```python
from build123d import *

# Parameters (mm, degrees)
F0_W         = 45
F0_H         = 45
F1_DEPTH     = 2
F2_R         = 8
F3_DEPTH     = 25
F4_W         = 23
F4_H         = 3.9995294809
F4_H_2       = 4
F5_DEPTH     = 9.8
F6_W         = 23
F6_H         = 9
F6_H_2       = 4
F7_DEPTH     = 2
F8_W         = 23
F8_H         = 13
F9_DEPTH     = 2
F10_W        = 2
F10_H        = 45
F11_DEPTH    = 7.7
F12_W        = 7
F12_H        = 45
F13_W        = 7
F13_H        = 45
F14_DEPTH    = 2
F15_T1_DEPTH = 23
F15_T3_DEPTH = 45


# Not quite as in the source:
# - a fillet or chamfer that OpenCascade refuses, or shapes differently, is made with other operations: its cross-section is extruded or revolved along the edge and cut away or added


with BuildPart() as f1:
    # F0 (on Top) → F1 (new body)
    with BuildSketch(Plane.XY):
        Rectangle(F0_W, F0_H)
    extrude(amount=F1_DEPTH)

    # F2 (on face) → F3 (cut)
    with BuildSketch(Plane.XY.offset(2)):
        Circle(F2_R)
    extrude(amount=-F3_DEPTH, mode=Mode.SUBTRACT)

    # F4 (on face) → F5 (join)
    with BuildSketch(Plane.XY.offset(2)):
        with Locations((0, 22.5)):
            Rectangle(F4_W, F4_H)
        with Locations((0, -22.5)):
            Rectangle(F4_W, F4_H_2)
    extrude(amount=-F5_DEPTH)

    # F6 (on face) → F7 (join)
    with BuildSketch(Plane(origin=(0, 0, -7.8), x_dir=(1, 0, 0), z_dir=(0, 0, -1))):
        with Locations((0, 16)):
            Rectangle(F6_W, F6_H)
        with Locations((0, 22.5)):
            Rectangle(F6_W, F6_H_2)
    extrude(amount=F7_DEPTH)

    # F8 (on face) → F9 (join)
    with BuildSketch(Plane(origin=(0, 0, -7.8), x_dir=(1, 0, 0), z_dir=(0, 0, -1))):
        with Locations((0, -17.9997647405)):
            Rectangle(F8_W, F8_H)
    extrude(amount=F9_DEPTH)

    # F10 (on face) → F11 (join)
    with BuildSketch(Plane(origin=(0, 0, 0), x_dir=(1, 0, 0), z_dir=(0, 0, -1))):
        with Locations((-21.5, 0)):
            Rectangle(F10_W, F10_H)
        with Locations((21.5, 0)):
            Rectangle(F10_W, F10_H)
    extrude(amount=F11_DEPTH)

    # F12 (on face) + F13 (on face) → F14 (join)
    with BuildSketch(Plane(origin=(0, 0, -7.7), x_dir=(1, 0, 0), z_dir=(0, 0, -1))):
        with Locations((-24, 0)):
            Rectangle(F12_W, F12_H)
    with BuildSketch(Plane(origin=(0, 0, -7.7), x_dir=(1, 0, 0), z_dir=(0, 0, -1))):
        with Locations((24, 0)):
            Rectangle(F13_W, F13_H)
    extrude(amount=F14_DEPTH)

    # F15: fillet of radius 5 on 8 edges, made by hand

    # F15_s2 → F15_t1 (join)
    with BuildSketch(Plane.YZ.offset(-11.5)):
        with BuildLine():
            ThreePointArc((-15.5, -7.8), (-19.0355339059, -6.3355339059), (-20.5, -2.8))
            Line((-20.5, -2.8), (-20.5, -7.8))
            Line((-20.5, -7.8), (-15.5, -7.8))
        make_face()
        with BuildLine():
            ThreePointArc((15.5002352595, -7.8), (19.0357691655, -6.3355339059), (20.5002352595, -2.8))
            Line((20.5002352595, -2.8), (20.5002352595, -7.8))
            Line((20.5002352595, -7.8), (15.5002352595, -7.8))
        make_face()
        with BuildLine():
            ThreePointArc((20.5002352595, -5), (19.0357691655, -1.4644660941), (15.5002352595, 0))
            Line((15.5002352595, 0), (20.5002352595, 0))
            Line((20.5002352595, 0), (20.5002352595, -5))
        make_face()
        with BuildLine():
            ThreePointArc((-20.5, -5), (-19.0355339059, -1.4644660941), (-15.5, 0))
            Line((-15.5, 0), (-20.5, 0))
            Line((-20.5, 0), (-20.5, -5))
        make_face()
    extrude(amount=F15_T1_DEPTH)

    # F15_s4 → F15_t3 (join)
    with BuildSketch(Plane.XZ.offset(-22.5)):
        with BuildLine():
            ThreePointArc((20.5, -5), (19.0355339059, -1.4644660941), (15.5, 0))
            Line((15.5, 0), (20.5, 0))
            Line((20.5, 0), (20.5, -5))
        make_face()
        with BuildLine():
            ThreePointArc((-20.5, -5), (-19.0355339059, -1.4644660941), (-15.5, 0))
            Line((-15.5, 0), (-20.5, 0))
            Line((-20.5, 0), (-20.5, -5))
        make_face()
        with BuildLine():
            ThreePointArc((-22.5, -2.7), (-23.9644660941, -6.2355339059), (-27.5, -7.7))
            Line((-27.5, -7.7), (-22.5, -7.7))
            Line((-22.5, -7.7), (-22.5, -2.7))
        make_face()
        with BuildLine():
            ThreePointArc((27.5, -7.7), (23.9644660941, -6.2355339059), (22.5, -2.7))
            Line((22.5, -2.7), (22.5, -7.7))
            Line((22.5, -7.7), (27.5, -7.7))
        make_face()
    extrude(amount=F15_T3_DEPTH)


solid = f1.part
```
Input: part model. Units: mm. Frame: model coordinates. A direction names the side the tool comes from. Give positions to 0.01 mm unless a question says otherwise; leave off trailing zeros. Order: outer loops, then holes, each group sorted by start corner. A loop starts at its lowest first (then second) coordinate and runs counter-clockwise, first axis right, second up.
1. Line query: probe 1 along X at (y, z) = (-13.5, -8); probe 2 along Z at (x, y) = (7, -15); probe 3 along Y at (x, z) = (0, 1.1). Output: solid intervals per line, ascending.
Computed:
probe 1: x = -27.5 to -20.5, -11.5 to 11.5, 20.5 to 27.5
probe 2: z = -9.8 to -7.8, 0 to 2
probe 3: y = -24.5 to -8, 8 to 24.5
2. Draft query along X for faces 1 (the face through (27.5, 0, -9)), 2 (the face through (0, 24.5, -4)), 3 (the face through (-23.93, 0.32, -6.2)), 4 (the face through (-19.07, 0.32, -1.5)). Return one class per face: released by +X, released by -X, zero draft, split by the parting line, or undercut.
Computed:
face 1: released by +X
face 2: zero draft
face 3: released by -X
face 4: undercut
3. Cut plane B-B (x = 0). Return loops of the section in (y, z).
Computed:
outline: (-24.5, -9.8) - (-11.5, -9.8) - (-11.5, -7.8) - (-15.5, -7.8) arc R5 cw to (-20.38, -3.9) arc R5 cw to (-15.5, 0) - (-8, 0) - (-8, 2) - (-24.5, 2) - close; (8, 0) - (15.5, 0) arc R5 cw to (20.38, -3.9) arc R5 cw to (15.5, -7.8) - (11.5, -7.8) - (11.5, -9.8) - (24.5, -9.8) - (24.5, 2) - (8, 2) - close
4. Set-up query: faces 5 (the face through (-21, 22.5, -3)), 6 (the face through (-22.5, 0, 0)), 7 (the face through (-0.161, 18.659, -1.125)), 8 (the face through (-24, 0, -9.7)), 9 (the face through (0, -11.5, -9)). Return all of +Z, -Z, +X, -X, +Y, -Y with unobstructed straight access to the full face (end or side cutting, diameter ignored); none if empty.
Computed:
face 5: +Z, -Z, -X, +Y
face 6: +Z, -X, +Y, -Y
face 7: none
face 8: -Z, -X, +Y, -Y
face 9: -Z
5. Cut plane C-C (z = -6.5). Return loops of the section in (x, y), and give its area (3 significant figures).
Computed:
outline: (-24.25, -22.5) - (-20.5, -22.5) - (-20.5, 22.5) - (-24.25, 22.5) - close; (-11.5, -24.5) - (11.5, -24.5) - (11.5, -18.86) - (-11.5, -18.86) - close; (-11.5, 18.86) - (11.5, 18.86) - (11.5, 24.5) - (-11.5, 24.5) - close; (20.5, -22.5) - (24.25, -22.5) - (24.25, 22.5) - (20.5, 22.5) - close
area: 597 mm2
6. Pin query (flat end, axial travel): pin 1 Ø4 at (y, z) = (-10.5, -1.5) entering from -X; pin 2 Ø6 at (y, z) = (-13.5, -1.5) entering from -X; pin 3 Ø6 at (x, y) = (21, -15.5) entering from -Z; pin 4 Ø14.5 at (x, y) = (0, 0) entering from -Z. Return the tip coordinate at first contact, or that it passes through.
Computed:
pin 1: stops at x = -22.56
pin 2: stops at x = -22.84
pin 3: stops at z = -9.7
pin 4: passes through
7. Cut plane A-A (y = 0). Return loops of the section in (x, z).
Computed:
outline: (-27.5, -9.7) - (-20.5, -9.7) - (-20.5, -5) arc R5 cw to (-15.5, 0) - (-8, 0) - (-8, 2) - (-22.5, 2) - (-22.5, -2.7) arc R5 cw to (-27.5, -7.7) - close; (8, 0) - (15.5, 0) arc R5 cw to (20.5, -5) - (20.5, -9.7) - (27.5, -9.7) - (27.5, -7.7) arc R5 cw to (22.5, -2.7) - (22.5, 2) - (8, 2) - close
8. Cut plane D-D (y = 10.5). Return loops of the section in (x, z).
Computed:
outline: (-27.5, -9.7) - (-20.5, -9.7) - (-20.5, -5) arc R5 cw to (-15.5, 0) - (15.5, 0) arc R5 cw to (20.5, -5) - (20.5, -9.7) - (27.5, -9.7) - (27.5, -7.7) arc R5 cw to (22.5, -2.7) - (22.5, 2) - (-22.5, 2) - (-22.5, -2.7) arc R5 cw to (-27.5, -7.7) - close
